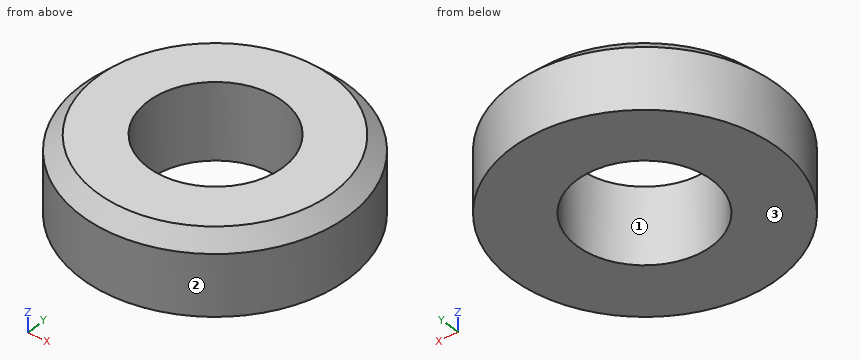
```python
from build123d import *

# Parameters (mm, degrees)
F0_R     = 44.395237
F1_DEPTH = 25.4
F2_SIZE  = 5.08
F3_R     = 22.466185
F4_DEPTH = 25.401


with BuildPart() as f1:
    # F0 (on Top) → F1 (new body)
    with BuildSketch(Plane.XY):
        with Locations((0, -24.399335)):
            Circle(F0_R)
    extrude(amount=F1_DEPTH)

    # F2
    f2_edges = [f1.edges().sort_by_distance(p)[0] for p in [
        (-44.395237, -24.399335, 25.4),
    ]]
    chamfer(f2_edges, length=F2_SIZE)

    # F3 (on Top) → F4 (cut, through all)
    with BuildSketch(Plane.XY):
        with Locations((0, -24.16065)):
            Circle(F3_R)
    extrude(amount=F4_DEPTH, mode=Mode.SUBTRACT)


solid = f1.part
```
Work out the finished part from the listing and answer in its coordinate system (mm). Face numbers are marked on the shaded views. Give positions to 0.01 mm unless a question says otherwise; leave off trailing zeros. Write each loop counter-clockwise with the first axis right and the second up, starting at its lowest first coordinate (ties: lowest second). Pieces come first, ordered by that corner, then holes. Notation, with made-up numbers: (82.25, 10.5) - (94.25, 10.5) arc R20 cw to (94.25, 29.5) - close; hole circle Ø1 at (-26.75, 71). An arc over 180 degrees is marked (long way). Use one line per item in the form item = value.
1. A cutting plane is placed at A-A (x = 0). Write down the section's boundary in (y, z), and give its area (3 significant figures).
Filled in:
outline = (-68.79, 0) - (-46.63, 0) - (-46.63, 25.4) - (-63.71, 25.4) - (-68.79, 20.32) - close; (-1.69, 0) - (20, 0) - (20, 20.32) - (14.92, 25.4) - (-1.69, 25.4) - close
area = 1,090 mm^2
2. Each of these flat-tipped pins is pushed along its axis until it touches: pin 1 Ø1.5 at (y, z) = (-57, 10.5) entering from -X; pin 2 Ø1.5 at (y, z) = (-57.5, 11.5) entering from -X; pin 3 Ø8 at (y, z) = (3, 11.5) entering from -X; pin 4 Ø2 at (x, y) = (-20.5, -28.5) entering from -Z. Where does it stop, or does it pass through?
Filled in:
pin_1 = -30.93
pin_2 = -30.4
pin_3 = -37.73
pin_4 = through
3. A cutting plane is placed at B-B (z = 18). Write down the section's boundary in (x, y).
Filled in:
outline = circle Ø88.79 at (0, -24.4); hole circle Ø44.93 at (0, -24.16)
4. Determine the mould class of the marked faces 1, 2 and 3 for opening direction X: released by +X, released by -X, zero draft, split by the parting line, or undercut.
Filled in:
face_1 = undercut
face_2 = split by the parting line
face_3 = zero draft
5. Consider L1, parallel to Y at x = 0, z = 9; L2, parallel to X at y = -23.5, z = 8.25; L3, parallel to X at y = -17, z = 13. Determine where each line is inside the solid, lowest interval first.
Filled in:
L1 = -68.79 to -46.63, -1.69 to 20
L2 = -44.39 to -22.46, 22.46 to 44.39
L3 = -43.77 to -21.29, 21.29 to 43.77
